```python
from build123d import *
from OCP.BRepFilletAPI import BRepFilletAPI_MakeChamfer

# Parameters (mm, degrees)
SKETCH_1_R          = 8
SKETCH_1_R_2        = 5
EXTRUDE_1_DEPTH     = 7.45
SKETCH_2_R          = 5
EXTRUDE_2_DEPTH     = 10
SKETCH_3_R          = 8
SKETCH_3_R_2        = 5
EXTRUDE_3_DEPTH     = 1.5
CHAMFER_1_SIZE      = 1
CHAMFER_1_SIZE2     = 0.577350269
SKETCH_1_2_R        = 8
CUT_EXTRUDE_1_DEPTH = 5.95


with BuildPart() as part:
    # Sketch 1 → Бобышка-Вытянуть1 (new body)
    with BuildSketch(Plane(origin=(0, 0, 0), x_dir=(1, 0, 0), z_dir=(0, 1, 0))):
        with Locations(Location((0, 0, 0), (0, 0, 270))):
            Circle(SKETCH_1_R)
        with Locations(Location((0, 0, 0), (0, 0, 270))):
            Circle(SKETCH_1_R_2, mode=Mode.SUBTRACT)
    extrude(amount=EXTRUDE_1_DEPTH)

    # Эскиз2 → Бобышка-Вытянуть2 (add)
    with BuildSketch(Plane(origin=(0, 7.45, 0), x_dir=(1, 0, 0), z_dir=(0, 1, 0))):
        with BuildLine():
            ThreePointArc((-2.557469435, 5.549004423), (-2.773881953, 5.444049863), (-2.985996064, 5.3306592))
            ThreePointArc((-2.985996064, 5.3306592), (-3.059404709, 5.231014138), (-3.032930262, 5.110113057))
            ThreePointArc((-3.032930262, 5.110113057), (-3.150528952, 4.33633109), (-3.922779328, 4.463599867))
            ThreePointArc((-3.922779328, 4.463599867), (-4.029582035, 4.526139051), (-4.14703464, 4.487115298))
            ThreePointArc((-4.14703464, 4.487115298), (-4.320422433, 4.320422433), (-4.487115298, 4.14703464))
            ThreePointArc((-4.487115298, 4.14703464), (-4.526139051, 4.029582035), (-4.463599867, 3.922779328))
            ThreePointArc((-4.463599867, 3.922779328), (-4.33633109, 3.150528952), (-5.110113057, 3.032930262))
            ThreePointArc((-5.110113057, 3.032930262), (-5.231014138, 3.059404709), (-5.3306592, 2.985996064))
            ThreePointArc((-5.3306592, 2.985996064), (-5.444049863, 2.773881953), (-5.549004423, 2.557469435))
            ThreePointArc((-5.549004423, 2.557469435), (-5.549823367, 2.433706366), (-5.457341217, 2.351456627))
            ThreePointArc((-5.457341217, 2.351456627), (-5.097662927, 1.65633109), (-5.797233315, 1.305376312))
            ThreePointArc((-5.797233315, 1.305376312), (-5.92039813, 1.293194518), (-5.992481697, 1.19258673))
            ThreePointArc((-5.992481697, 1.19258673), (-6.034775761, 0.955814581), (-6.067718334, 0.717561302))
            ThreePointArc((-6.067718334, 0.717561302), (-6.030252304, 0.599602562), (-5.916879985, 0.549956967))
            ThreePointArc((-5.916879985, 0.549956967), (-5.36, 0), (-5.916879985, -0.549956967))
            ThreePointArc((-5.916879985, -0.549956967), (-6.030252304, -0.599602562), (-6.067718334, -0.717561302))
            ThreePointArc((-6.067718334, -0.717561302), (-6.034775761, -0.955814581), (-5.992481697, -1.19258673))
            ThreePointArc((-5.992481697, -1.19258673), (-5.92039813, -1.293194518), (-5.797233315, -1.305376312))
            ThreePointArc((-5.797233315, -1.305376312), (-5.097662927, -1.65633109), (-5.457341217, -2.351456627))
            ThreePointArc((-5.457341217, -2.351456627), (-5.549823367, -2.433706366), (-5.549004423, -2.557469435))
            ThreePointArc((-5.549004423, -2.557469435), (-5.444049863, -2.773881953), (-5.3306592, -2.985996064))
            ThreePointArc((-5.3306592, -2.985996064), (-5.231014138, -3.059404709), (-5.110113057, -3.032930262))
            ThreePointArc((-5.110113057, -3.032930262), (-4.33633109, -3.150528952), (-4.463599867, -3.922779328))
            ThreePointArc((-4.463599867, -3.922779328), (-4.526139051, -4.029582035), (-4.487115298, -4.14703464))
            ThreePointArc((-4.487115298, -4.14703464), (-4.320422433, -4.320422433), (-4.14703464, -4.487115298))
            ThreePointArc((-4.14703464, -4.487115298), (-4.029582035, -4.526139051), (-3.922779328, -4.463599867))
            ThreePointArc((-3.922779328, -4.463599867), (-3.150528952, -4.33633109), (-3.032930262, -5.110113057))
            ThreePointArc((-3.032930262, -5.110113057), (-3.059404709, -5.231014138), (-2.985996064, -5.3306592))
            ThreePointArc((-2.985996064, -5.3306592), (-2.773881953, -5.444049863), (-2.557469435, -5.549004423))
            ThreePointArc((-2.557469435, -5.549004423), (-2.433706366, -5.549823367), (-2.351456627, -5.457341217))
            ThreePointArc((-2.351456627, -5.457341217), (-1.65633109, -5.097662927), (-1.305376312, -5.797233315))
            ThreePointArc((-1.305376312, -5.797233315), (-1.293194518, -5.92039813), (-1.19258673, -5.992481697))
            ThreePointArc((-1.19258673, -5.992481697), (-0.955814581, -6.034775761), (-0.717561302, -6.067718334))
            ThreePointArc((-0.717561302, -6.067718334), (-0.599602562, -6.030252304), (-0.549956967, -5.916879985))
            ThreePointArc((-0.549956967, -5.916879985), (0, -5.36), (0.549956967, -5.916879985))
            ThreePointArc((0.549956967, -5.916879985), (0.599602562, -6.030252304), (0.717561302, -6.067718334))
            ThreePointArc((0.717561302, -6.067718334), (0.955814581, -6.034775761), (1.19258673, -5.992481697))
            ThreePointArc((1.19258673, -5.992481697), (1.293194518, -5.92039813), (1.305376312, -5.797233315))
            ThreePointArc((1.305376312, -5.797233315), (1.65633109, -5.097662927), (2.351456627, -5.457341217))
            ThreePointArc((2.351456627, -5.457341217), (2.433706366, -5.549823367), (2.557469435, -5.549004423))
            ThreePointArc((2.557469435, -5.549004423), (2.773881953, -5.444049863), (2.985996064, -5.3306592))
            ThreePointArc((2.985996064, -5.3306592), (3.059404709, -5.231014138), (3.032930262, -5.110113057))
            ThreePointArc((3.032930262, -5.110113057), (3.150528952, -4.33633109), (3.922779328, -4.463599867))
            ThreePointArc((3.922779328, -4.463599867), (4.029582035, -4.526139051), (4.14703464, -4.487115298))
            ThreePointArc((4.14703464, -4.487115298), (4.320422433, -4.320422433), (4.487115298, -4.14703464))
            ThreePointArc((4.487115298, -4.14703464), (4.526139051, -4.029582035), (4.463599867, -3.922779328))
            ThreePointArc((4.463599867, -3.922779328), (4.33633109, -3.150528952), (5.110113057, -3.032930262))
            ThreePointArc((5.110113057, -3.032930262), (5.231014138, -3.059404709), (5.3306592, -2.985996064))
            ThreePointArc((5.3306592, -2.985996064), (5.444049863, -2.773881953), (5.549004423, -2.557469435))
            ThreePointArc((5.549004423, -2.557469435), (5.549823367, -2.433706366), (5.457341217, -2.351456627))
            ThreePointArc((5.457341217, -2.351456627), (5.097662927, -1.65633109), (5.797233315, -1.305376312))
            ThreePointArc((5.797233315, -1.305376312), (5.92039813, -1.293194518), (5.992481697, -1.19258673))
            ThreePointArc((5.992481697, -1.19258673), (6.034775761, -0.955814581), (6.067718334, -0.717561302))
            ThreePointArc((6.067718334, -0.717561302), (6.030252304, -0.599602562), (5.916879985, -0.549956967))
            ThreePointArc((5.916879985, -0.549956967), (5.36, 0), (5.916879985, 0.549956967))
            ThreePointArc((5.916879985, 0.549956967), (6.030252304, 0.599602562), (6.067718334, 0.717561302))
            ThreePointArc((6.067718334, 0.717561302), (6.034775761, 0.955814581), (5.992481697, 1.19258673))
            ThreePointArc((5.992481697, 1.19258673), (5.92039813, 1.293194518), (5.797233315, 1.305376312))
            ThreePointArc((5.797233315, 1.305376312), (5.097662927, 1.65633109), (5.457341217, 2.351456627))
            ThreePointArc((5.457341217, 2.351456627), (5.549823367, 2.433706366), (5.549004423, 2.557469435))
            ThreePointArc((5.549004423, 2.557469435), (5.444049863, 2.773881953), (5.3306592, 2.985996064))
            ThreePointArc((5.3306592, 2.985996064), (5.231014138, 3.059404709), (5.110113057, 3.032930262))
            ThreePointArc((5.110113057, 3.032930262), (4.33633109, 3.150528952), (4.463599867, 3.922779328))
            ThreePointArc((4.463599867, 3.922779328), (4.526139051, 4.029582035), (4.487115298, 4.14703464))
            ThreePointArc((4.487115298, 4.14703464), (4.320422433, 4.320422433), (4.14703464, 4.487115298))
            ThreePointArc((4.14703464, 4.487115298), (4.029582035, 4.526139051), (3.922779328, 4.463599867))
            ThreePointArc((3.922779328, 4.463599867), (3.150528952, 4.33633109), (3.032930262, 5.110113057))
            ThreePointArc((3.032930262, 5.110113057), (3.059404709, 5.231014138), (2.985996064, 5.3306592))
            ThreePointArc((2.985996064, 5.3306592), (2.773881953, 5.444049863), (2.557469435, 5.549004423))
            ThreePointArc((2.557469435, 5.549004423), (2.433706366, 5.549823367), (2.351456627, 5.457341217))
            ThreePointArc((2.351456627, 5.457341217), (1.65633109, 5.097662927), (1.305376312, 5.797233315))
            ThreePointArc((1.305376312, 5.797233315), (1.293194518, 5.92039813), (1.19258673, 5.992481697))
            ThreePointArc((1.19258673, 5.992481697), (0.955814581, 6.034775761), (0.717561302, 6.067718334))
            ThreePointArc((0.717561302, 6.067718334), (0.599602562, 6.030252304), (0.549956967, 5.916879985))
            ThreePointArc((0.549956967, 5.916879985), (0, 5.36), (-0.549956967, 5.916879985))
            ThreePointArc((-0.549956967, 5.916879985), (-0.599602562, 6.030252304), (-0.717561302, 6.067718334))
            ThreePointArc((-0.717561302, 6.067718334), (-0.955814581, 6.034775761), (-1.19258673, 5.992481697))
            ThreePointArc((-1.19258673, 5.992481697), (-1.293194518, 5.92039813), (-1.305376312, 5.797233315))
            ThreePointArc((-1.305376312, 5.797233315), (-1.65633109, 5.097662927), (-2.351456627, 5.457341217))
            ThreePointArc((-2.351456627, 5.457341217), (-2.433706366, 5.549823367), (-2.557469435, 5.549004423))
        make_face()
        with Locations(Location((0, 0, 0), (0, 0, 270))):
            Circle(SKETCH_2_R, mode=Mode.SUBTRACT)
    extrude(amount=EXTRUDE_2_DEPTH)

    # Эскиз3 → Бобышка-Вытянуть3 (add)
    with BuildSketch(Plane(origin=(0, 17.45, 0), x_dir=(1, 0, 0), z_dir=(0, 1, 0))):
        with Locations(Location((0, 0, 0), (0, 0, 270))):
            Circle(SKETCH_3_R)
        with Locations(Location((0, 0, 0), (0, 0, 270))):
            Circle(SKETCH_3_R_2, mode=Mode.SUBTRACT)
    extrude(amount=EXTRUDE_3_DEPTH)

    # Фаска1: one chamfer whose edges measure the first distance from different faces: ONE call of the kernel's chamfer builder (chamfer() names one face for all edges)
    chamfer_1_edges_1 = [part.edges().sort_by_distance(p)[0] for p in [
        (0, 17.45, -8),
    ]]
    chamfer_1_side_1 = [part.faces().sort_by_distance(p)[0] for p in [
        (0, 17.45, -7.77372583),
    ]]
    chamfer_1_edges_2 = [part.edges().sort_by_distance(p)[0] for p in [
        (0, 7.45, -8),
    ]]
    chamfer_1_side_2 = [part.faces().sort_by_distance(p)[0] for p in [
        (0, 7.45, -7.77372583),
    ]]
    chamfer_1 = BRepFilletAPI_MakeChamfer(part.part.solid().wrapped)
    for e in chamfer_1_edges_1:
        chamfer_1.Add(CHAMFER_1_SIZE, CHAMFER_1_SIZE2, e.wrapped, chamfer_1_side_1[0].wrapped)  # the first distance lies on this face
    for e in chamfer_1_edges_2:
        chamfer_1.Add(CHAMFER_1_SIZE, CHAMFER_1_SIZE2, e.wrapped, chamfer_1_side_2[0].wrapped)  # the first distance lies on this face
    add(Compound.cast(chamfer_1.Shape()), mode=Mode.REPLACE)

    # Sketch 1 2 → 切除-拉伸1 (cut)
    with BuildSketch(Plane.XZ):
        with Locations(Location((0, 0, 0), (0, 0, 270))):
            Circle(SKETCH_1_2_R)
    extrude(amount=-CUT_EXTRUDE_1_DEPTH, mode=Mode.SUBTRACT)


solid = part.part
```
Input: part model. Units: mm. Frame: model coordinates. A direction names the side the tool comes from. Give positions to 0.01 mm unless a question says otherwise; leave off trailing zeros. Write each loop counter-clockwise with the first axis right and the second up, starting at its lowest first coordinate (ties: lowest second). Pieces come first, ordered by that corner, then holes. Notation, with made-up numbers: (32, -29) - (42, -29) arc R15 ccw to (42, -3) - close; hole circle Ø9 at (8, -1.5). An arc over 180 degrees is marked (long way). Write item = value, one per line. Start each with the question number.
1. Access query for faces 1 (the flat face through (-4.63, 17.45, -3.14)), 2 (the cylindrical face through (-7.81, 6.4, -1.73)). Directions: +Z, -Z, +X, -X, +Y, -Y. A direction counts if a zero-diameter tool reaches every point of the face in a straight line with its end or side. Return the directions, or none.
2. Section query A-A, the plane x = 0. Output: boundary loops of the cut face in (y, z), then the cut area to 3 significant figures.
3. Ray query, L1, parallel to Y at x = -6, z = 3.5; L2, parallel to Z at x = 0.75, y = 6.75. Return the intervals inside material, ascending.
4. First-contact query: pin 1 Ø6 at (y, z) = (9.5, 6.5) entering from +X; pin 2 Ø1.5 at (x, z) = (3.5, 3) entering from +Y; pin 3 Ø2 at (y, z) = (16.5, 3) entering from -X; pin 4 Ø2 at (y, z) = (7.5, 4.5) entering from +X. Flat tips, straight axial feed; report the tip coordinate or a pass-through.
5. Section query B-B, the plane z = 0. Output: boundary loops of the cut face in (x, y), then the cut area to 3 significant figures.
6. Mould query, pull axis Z, two halves, no side actions, for faces 3 (the cylindrical face through (-4.33, 12.38, -3.16)), 4 (the flat face through (-5.2, 5.95, 0.1)), 5 (the cylindrical face through (-7.81, 18.48, -1.73)), 6 (the cylindrical face through (-4.344, 12.38, 3.141)). Classes: released by +Z, released by -Z, zero draft, split by the parting line, or undercut.
Check sheet entries:
q1.face_1 = none
q1.face_2 = +Y, -Y
q2.outline = (5.95, -8) - (6.87, -8) - (7.45, -7) - (7.45, -5.36) - (17.45, -5.36) - (17.45, -7) - (18.03, -8) - (18.95, -8) - (18.95, -5) - (5.95, -5) - close; (5.95, 5) - (18.95, 5) - (18.95, 8) - (18.03, 8) - (17.45, 7) - (17.45, 5.36) - (7.45, 5.36) - (7.45, 7) - (6.87, 8) - (5.95, 8) - close
q2.area = 24.0 mm2
q3.L1 = 5.95 to 7.45, 17.45 to 18.95
q3.L2 = -7.96 to -4.94, 4.94 to 7.96
q4.pin_1 = 6.2
q4.pin_2 = 18.95
q4.pin_3 = -6.47
q4.pin_4 = 7.08
q5.outline = (-8, 5.95) - (-5, 5.95) - (-5, 18.95) - (-8, 18.95) - (-8, 18.03) - (-7, 17.45) - (-5.36, 17.45) - (-5.36, 7.45) - (-7, 7.45) - (-8, 6.87) - close; (5, 5.95) - (8, 5.95) - (8, 6.87) - (7, 7.45) - (5.36, 7.45) - (5.36, 17.45) - (7, 17.45) - (8, 18.03) - (8, 18.95) - (5, 18.95) - close
q5.area = 24.0 mm2
q6.face_3 = undercut
q6.face_4 = zero draft
q6.face_5 = split by the parting line
q6.face_6 = undercut
